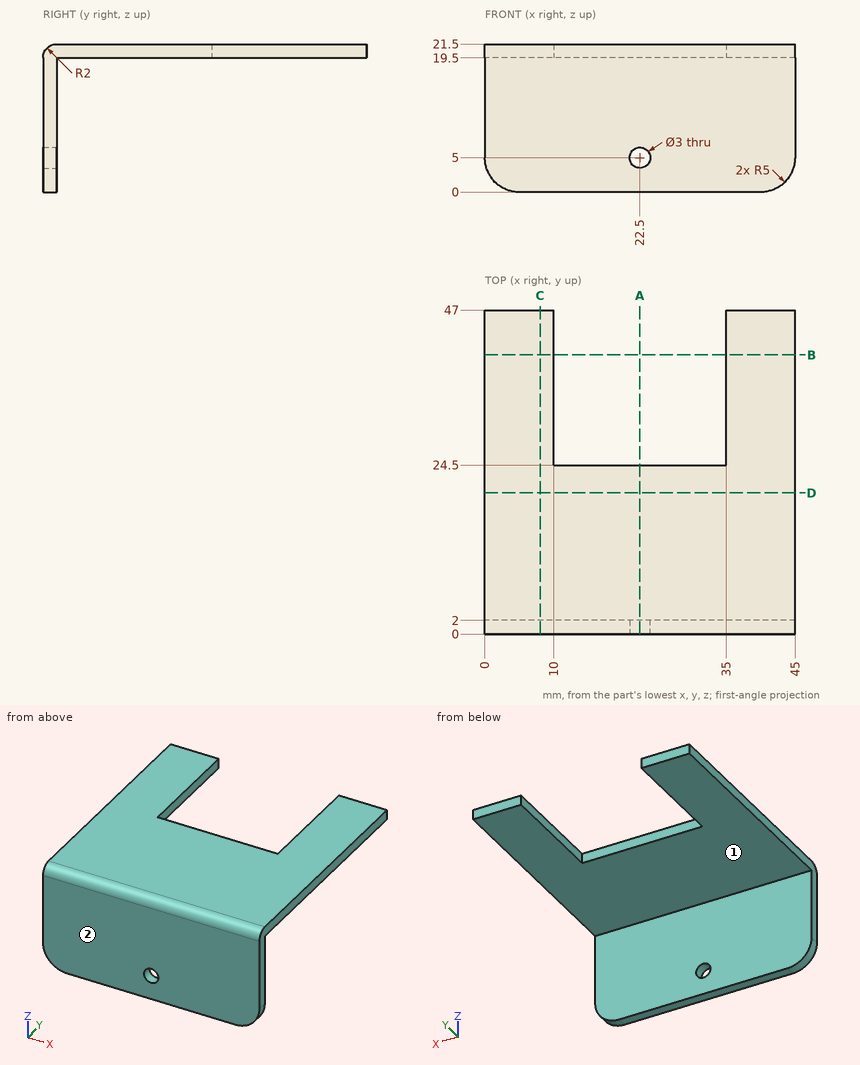
Print and shaded views of the part. All mm, measured from the part's lowest x, y and z. A direction names the side the tool comes from. Coordinates: 2 decimals unless noted, no trailing zeros. Order: outer loops, then holes, each group sorted by start corner. A loop starts at its lowest first (then second) coordinate and runs counter-clockwise, first axis right, second up.
Item 1: Saw through at D-D on y = 20.5. List the corners of the cut face in (x, z).
Filled in:
outline: (0, 19.5) - (45, 19.5) - (45, 21.5) - (0, 21.5) - close
Item 2: Saw through at C-C on x = 8. List the corners of the cut face in (y, z), then the cut area to 3 significant figures.
Filled in:
outline: (0, 0) - (2, 0) - (2, 19.5) - (47, 19.5) - (47, 21.5) - (2, 21.5) arc R2 ccw to (0, 19.5) - close
area: 132 mm2
Item 3: Drill centre lines: L1, parallel to Y at x = 9.5, z = 13; L2, parallel to Z at x = 34, y = 21; L3, parallel to Z at x = 22.5, y = 1.05. Where is each one in solid material? Low to high.
Filled in:
L1: y = 0 to 2
L2: z = 19.5 to 21.5
L3: z = 0 to 3.5, 6.5 to 21.26
Item 4: Saw through at A-A on x = 22.5. List the corners of the cut face in (y, z).
Filled in:
outline: (0, 0) - (2, 0) - (2, 3.5) - (0, 3.5) - close; (0, 6.5) - (2, 6.5) - (2, 19.5) - (24.5, 19.5) - (24.5, 21.5) - (2, 21.5) arc R2 ccw to (0, 19.5) - close
Item 5: Saw through at B-B on y = 40.5. List the corners of the cut face in (x, z), then the cut area to 3 significant figures.
Filled in:
outline: (0, 19.5) - (10, 19.5) - (10, 21.5) - (0, 21.5) - close; (35, 19.5) - (45, 19.5) - (45, 21.5) - (35, 21.5) - close
area: 40.0 mm2
Item 6: Tool access for the marked faces 1 and 2: list every direction of +Z, -Z, +X, -X, +Y, -Y with a clear straight run to the whole face (end or side of a thin tool).
Filled in:
face 1: -Z, +X, -X, +Y
face 2: +Z, -Z, +X, -X, -Y
Item 7: Drop flat-ended pins along their axis: pin 1 Ø5 at (y, z) = (27, 18) entering from +X; pin 2 Ø4 at (x, y) = (40.5, 7) entering from -Z; pin 3 Ø1 at (x, z) = (18.5, 14.5) entering from +Y; pin 4 Ø1.6 at (x, z) = (17.5, 20.5) entering from +Y. Give the stop position or say it passes through.
Filled in:
pin 1: stops at x = 45
pin 2: stops at z = 19.5
pin 3: stops at y = 2
pin 4: stops at y = 24.5
